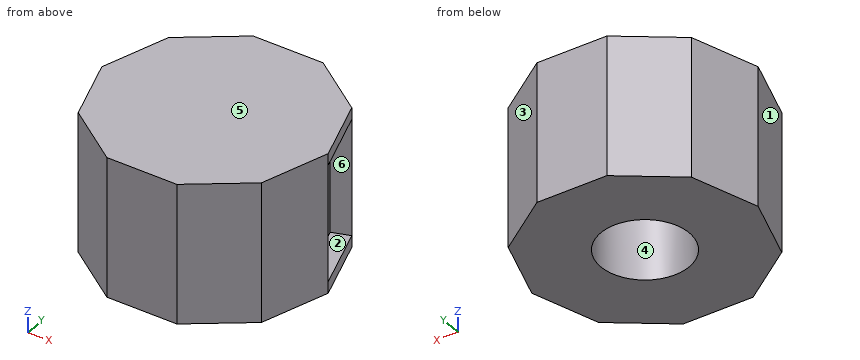
```python
from build123d import *

# Parameters (mm, degrees)
F1_DEPTH = 76.2
F2_R     = 24.13
F3_DEPTH = 33.02
F4_W     = 38.1
F4_H     = 63.5
F5_DEPTH = 10.16


with BuildPart() as f1:
    # F0 (on Top) → F1 (new body)
    with BuildSketch(Plane.XY):
        Polygon((19.05, 58.6298713832), (-19.05, 58.6298713832), (-49.8735474857, 36.2352532708), (-61.6470949714, 0), (-49.8735474857, -36.2352532708), (-19.05, -58.6298713832), (19.05, -58.6298713832), (49.8735474857, -36.2352532708), (61.6470949714, 0), (49.8735474857, 36.2352532708), align=None)
    extrude(amount=F1_DEPTH)

    # F2 (on face) → F3 (cut)
    with BuildSketch(Plane(origin=(0, 0, 0), x_dir=(1, 0, 0), z_dir=(0, 0, -1))):
        Circle(F2_R)
    extrude(amount=-F3_DEPTH, mode=Mode.SUBTRACT)

    # F4 (on face) → F5 (cut)
    with BuildSketch(Plane(origin=(55.7603212285, 18.1176266354, 0), x_dir=(-0.3090169944, 0.9510565163, 0), z_dir=(0.9510565163, 0.3090169944, 0))):
        with Locations((0, 38.1)):
            Rectangle(F4_W, F4_H)
    extrude(amount=-F5_DEPTH, mode=Mode.SUBTRACT)


solid = f1.part
```
The model under review builds one solid part; all positions refer to its coordinate system, in mm. Face numbers are marked on the shaded views. A direction names the side the tool comes from. Coordinates: 2 decimals unless noted, no trailing zeros. Order: outer loops, then holes, each group sorted by start corner. A loop starts at its lowest first (then second) coordinate and runs counter-clockwise, first axis right, second up. Notation, with made-up numbers: (66.25, 77.5) -> (124.25, 77.5) arc R31 ccw to (124.25, 115.5) -> close; hole circle Ø7 at (55, 35.5). An arc over 180 degrees is marked (long way). Answer in a Markdown table with one row per item. Add a question column.
Item 1: We need section C-C on z = 18.5. Write out the cut boundary in (x, y), plus the area to 3 significant figures.
Item 2: We need section B-B on x = 0. Write out the cut boundary in (y, z).
Item 3: Clearance check with flat-ended pins moving along their axes: pin 1 (4 mm diameter, centred on x = -37.5, z = 49.5, fed in from -Y); pin 2 (5 mm diameter, centred on y = -12.5, z = 29, fed in from +X); pin 3 (1 mm diameter, centred on y = 42.5, z = 38.5, fed in from -X). State where each tip first meets the part, or that it passes through.
Item 4: We need section A-A on z = 40.5. Write out the cut boundary in (x, y).
Item 5: We need section D-D on y = 9. Write out the cut boundary in (x, z), plus the area to 3 significant figures.
Item 6: To check wall thickness, follow probe 1 along Y at (x, z) = (0, 8); probe 2 along Z at (x, y) = (-6, -12.5); probe 3 along Y at (x, z) = (-20.5, 19.5). State the ranges of each line that lie inside material, in increasing order.
Item 7: Machinability: for the marked faces 4, 5 and 6, which of the approach directions +Z, -Z, +X, -X, +Y, -Y give a long, thin tool a straight path to every point of the face, cutting with its end or side? Answer none if there is none.
Item 8: Mouldability with a two-part tool opening along Y and no side actions: class the marked faces 1, 2 and 3 as +Y half, -Y half, draft (parallel to the pull), parting line (faces both ways), or undercut.
Final values:
| question | item | result |
|---|---|---|
| 1 | outline | (-61.65, 0) -> (-49.87, -36.24) -> (-19.05, -58.63) -> (19.05, -58.63) -> (49.87, -36.24) -> (61.65, 0) -> (51.98, -3.14) -> (40.21, 33.1) -> (49.87, 36.24) -> (19.05, 58.63) -> (-19.05, 58.63) -> (-49.87, 36.24) -> close; hole circle Ø48.26 at (0, 0) |
| 1 | area | 8,950 mm2 |
| 2 | outline | (-58.63, 0) -> (-24.13, 0) -> (-24.13, 33.02) -> (24.13, 33.02) -> (24.13, 0) -> (58.63, 0) -> (58.63, 76.2) -> (-58.63, 76.2) -> close |
| 3 | pin 1 | stops at y = -46.68 |
| 3 | pin 2 | stops at x = 58.4 |
| 3 | pin 3 | stops at x = -41.94 |
| 4 | outline | (-61.65, 0) -> (-49.87, -36.24) -> (-19.05, -58.63) -> (19.05, -58.63) -> (49.87, -36.24) -> (61.65, 0) -> (51.98, -3.14) -> (40.21, 33.1) -> (49.87, 36.24) -> (19.05, 58.63) -> (-19.05, 58.63) -> (-49.87, 36.24) -> close |
| 5 | outline | (-58.72, 0) -> (-22.39, 0) -> (-22.39, 33.02) -> (22.39, 33.02) -> (22.39, 0) -> (58.72, 0) -> (58.72, 6.35) -> (48.04, 6.35) -> (48.04, 69.85) -> (58.72, 69.85) -> (58.72, 76.2) -> (-58.72, 76.2) -> close |
| 5 | area | 6,790 mm2 |
| 6 | probe 1 | y = -58.63 to -24.13, 24.13 to 58.63 |
| 6 | probe 2 | z = 33.02 to 76.2 |
| 6 | probe 3 | y = -57.58 to -12.73, 12.73 to 57.58 |
| 7 | face 4 | -Z |
| 7 | face 5 | +Z, +X, -X, +Y, -Y |
| 7 | face 6 | +X |
| 8 | face 1 | -Y half |
| 8 | face 2 | undercut |
| 8 | face 3 | +Y half |
